Autodesk Inventor part; units mm, degrees
ref_plane "YZ Plane" through (0, 0, 0) normal (1, 0, 0) x (0, 1, 0)
ref_plane "XZ Plane" through (0, 0, 0) normal (0, 1, 0) x (-1, 0, 0)
ref_plane "XY Plane" through (0, 0, 0) normal (0, 0, 1) x (1, 0, 0)
sketch "Sketch1" plane through (0, 0, 0) normal (0, 0, 1) x (1, 0, 0)
  line L0 (-3.175, -3.175) -> (3.175, -3.175)
  line L1 (3.175, -3.175) -> (3.175, 3.175)
  line L2 (3.175, 3.175) -> (-3.175, 3.175)
  line L3 (-3.175, 3.175) -> (-3.175, -3.175)
  line L4 (-3.175, -3.175) -> (3.175, 3.175) construction
  line L5 (3.175, -3.175) -> (-3.175, 3.175) construction
  circle A0 centre (0, 0) radius 3.81
  point P0 (2.1061, -3.175)
  point P1 (3.175, -2.1061)
  point P2 (3.175, 2.1061)
  point P3 (2.1061, 3.175)
  point P4 (-2.1061, 3.175)
  point P5 (-3.175, 2.1061)
  point P6 (-3.175, -2.1061)
  point P7 (-2.1061, -3.175)
  dimension "d0" = 7.62
  dimension "d1" = 6.35
extrude "Extrusion1" add sketch "Sketch1" against normal blind 12.7 contours A0 L3 L2 L1 L0
sketch "Sketch2" plane through (0, 0, 0) normal (0, 0, 1) x (1, 0, 0)
  arc A0 (2.1061, -3.175) -> (3.175, -2.1061) centre (0, 0) ccw construction
  circle A1 centre (0, 0) radius 2.1082
  dimension "d4" = 4.2164
extrude "Extrusion2" cut sketch "Sketch2" against normal blind 12.7
fillet "Fillet1" radius 0.254 8 edges at (2.1061, 3.175, -6.35) (3.175, 2.1061, -6.35) (3.175, -2.1061, -6.35) (2.1061, -3.175, -6.35) (-2.1061, -3.175, -6.35) (-3.175, -2.1061, -6.35) (-3.175, 2.1061, -6.35) (-2.1061, 3.175, -6.35)
chamfer "Chamfer1" distance 0.7937 angle 45 2 edges at (-2.1082, 0, 0) (-2.1082, 0, -12.7)
properties part number "HS Shaft Adapter Circle"
Can you work these out from the model? Positions are in its coordinate system, mm. Give positions to 0.01 mm unless a question says otherwise; leave off trailing zeros. Loops run counter-clockwise (first coordinate to the right, second up) from the corner with the lowest first, then second, coordinate; pieces in that order, holes last. Notation, with made-up numbers: M -19,-35.75 L -8,-35.75 A20 cw -8,-10.75 Z; hole C 26.5,1.5 d9. An arc over 180 degrees is marked long. Answer in a Markdown table with one row per item.
1. Suppose I cut it at A-A on y = 0. Write out the boundary of the cut face in (x, z) (3 decimals).
Taken from the geometry:
| item | result |
|---|---|
| outline | M -3.175,-12.7 L -2.902,-12.7 L -2.108,-11.906 L -2.108,-0.794 L -2.902,0 L -3.175,0 Z; M 2.108,-11.906 L 2.902,-12.7 L 3.175,-12.7 L 3.175,0 L 2.902,0 L 2.108,-0.794 Z |
2. Thinking about a two-plate mould opening in X: for faces 1 (the flat face through (-1, 3, 0)), 2 (the cylindrical face through (2.7, 2.69, -6.26)), 3 (the cylindrical face through (-0.27, 2.09, -6.27)), which applies, released by +X, released by -X, zero draft, split by the parting line, or undercut?
Taken from the geometry:
| item | result |
|---|---|
| face 1 | zero draft |
| face 2 | released by +X |
| face 3 | undercut |
3. Suppose I cut it at B-B on z = -6. Write out the boundary of the cut face in (x, y) (3 decimals), plus the area to 3 significant figures.
Taken from the geometry:
| item | result |
|---|---|
| outline | M -3.175,-2.028 A0.254 ccw -3.13,-2.173 A3.81 ccw -2.173,-3.13 A0.254 ccw -2.028,-3.175 L 2.028,-3.175 A0.254 ccw 2.173,-3.13 A3.81 ccw 3.13,-2.173 A0.254 ccw 3.175,-2.028 L 3.175,2.028 A0.254 ccw 3.13,2.173 A3.81 ccw 2.173,3.13 A0.254 ccw 2.028,3.175 L -2.028,3.175 A0.254 ccw -2.173,3.13 A3.81 ccw -3.13,2.173 A0.254 ccw -3.175,2.028 Z; hole C 0,0 d4.216 |
| area | 24.4 mm² |
4. If I drill on line 1 along Y through (x, z) = (0, -8.75) (3 decimals); line 2 along Y through (x, z) = (1, -5.5) (3 decimals); line 3 along X through (y, z) = (-0.25, -0.5) (3 decimals), over which ranges is the centre line in solid material (lowest first)?
Taken from the geometry:
| item | result |
|---|---|
| line 1 | y = -3.175 to -2.108, 2.108 to 3.175 |
| line 2 | y = -3.175 to -1.856, 1.856 to 3.175 |
| line 3 | x = -3.175 to -2.389, 2.389 to 3.175 |
